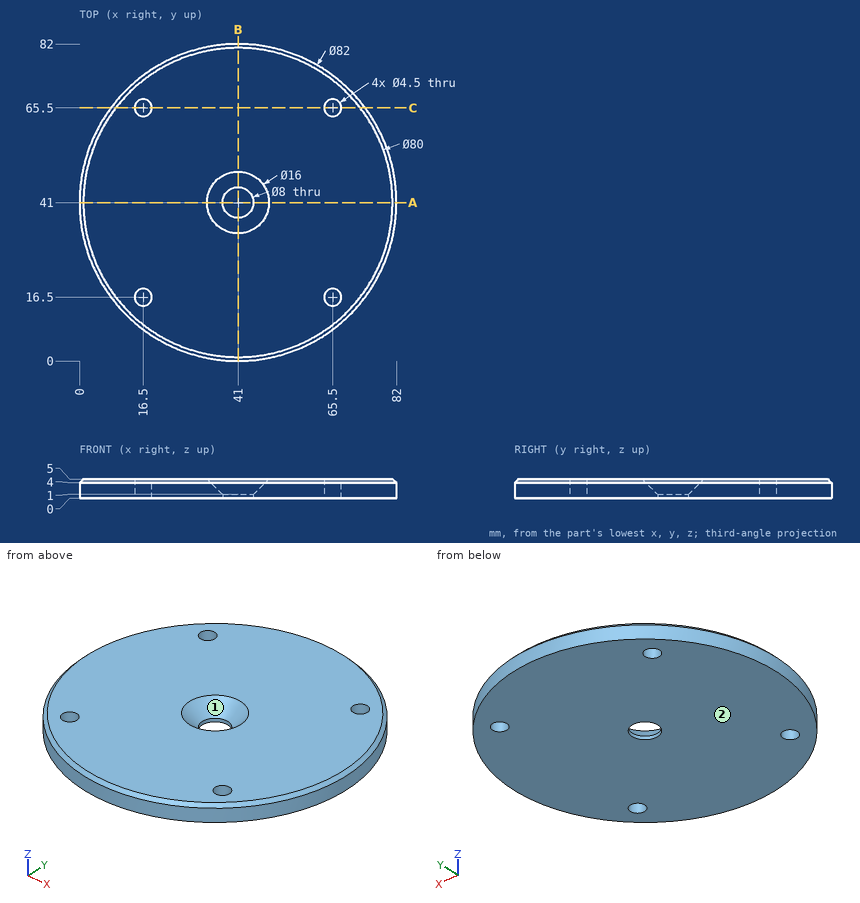
Job drawing, mm, ordinate dimensions from the low corner. One solid piece. Give positions to 0.01 mm unless a question says otherwise; leave off trailing zeros. Write each loop counter-clockwise with the first axis right and the second up, starting at its lowest first coordinate (ties: lowest second). Pieces come first, ordered by that corner, then holes. Notation, with made-up numbers: M 6.5,-14 L 44.5,-14 A25 cw 44.5,17 Z; hole C 57,15 d6. An arc over 180 degrees is marked long. One line per item, written item: value. Start each with the question number.
Q1. Saw through at A-A, the plane y = 41. Write the cut outline in (x, z).
Q2. Saw through at C-C, the plane y = 65.5. State how many separate pieces and enclosed holes the cut face has, plus the area to 3 significant figures.
Q3. Two-plate mould, pull along X, no slides. Class the marked faces 1 and 2: +X half, -X half, draft (parallel to the pull), parting line (faces both ways), or undercut.
Q4. Probe probe 1 along Y at (x, z) = (41, 0.35); probe 2 along Y at (x, z) = (65.5, 3.95); probe 3 along Y at (x, z) = (16, 1.25). List the from-to ranges inside material, lowest first. Write a range as [from, to].
Q5. Drop flat-ended pins along their axis: pin 1 Ø3 at (y, z) = (28.5, 4) entering from -X; pin 2 Ø1.5 at (x, z) = (61, 3) entering from -Y; pin 3 Ø1.5 at (x, z) = (9.5, 0.5) entering from -Y. Give the stop position or say it passes through.
Output values:
1. outline: M 0,0 L 37,0 L 37,1 L 33,5 L 1,5 L 0,4 Z; M 45,0 L 82,0 L 82,4 L 81,5 L 49,5 L 45,1 Z
2. separate pieces: 3
2. enclosed holes: 0
2. area: 282 mm²
3. face 1: undercut
3. face 2: draft
4. probe 1: y = [0, 37], [45, 82]
4. probe 2: y = [8.13, 14.25], [18.75, 63.25], [67.75, 73.87]
4. probe 3: y = [8.5, 14.31], [18.69, 63.31], [67.69, 73.5]
5. pin 1: stops at x = 1.5
5. pin 2: stops at y = 4.8
5. pin 3: stops at y = 13.88
